from build123d import *

# Parameters (mm, degrees)
SKETCH1_R           = 10
BOSS_EXTRUDE1_DEPTH = 10


with BuildPart() as part:
    # Sketch1 → Boss-Extrude1 (new body)
    with BuildSketch(Plane.XY):
        Polygon((322.382476836, -17.859318996), (322.382476836, 42.140681004), (371.94488009, 42.140681004), (371.94488009, 332.140681004), (277.025034275, 332.140681004), (169.187054595, 271.975052979), (169.187054595, 205.170044114), (169.187054595, -17.859318996), align=None)
        with Locations((229.870255563, 265.671146953)):
            Circle(SKETCH1_R, mode=Mode.SUBTRACT)
        with Locations((229.870255563, 102.825256229)):
            Circle(SKETCH1_R, mode=Mode.SUBTRACT)
        with Locations((340.159565259, 299.323240315)):
            Circle(SKETCH1_R, mode=Mode.SUBTRACT)
        with Locations((340.159565259, 67.667528684)):
            Circle(SKETCH1_R, mode=Mode.SUBTRACT)
        with BuildLine():
            Line((312.226028305, 265.671146953), (312.226028305, 115.671146953))
            ThreePointArc((312.226028305, 115.671146953), (288.591642629, 92.036761277), (264.957256952, 115.671146953))
            Line((264.957256952, 115.671146953), (264.957256952, 265.671146953))
            ThreePointArc((264.957256952, 265.671146953), (288.591642629, 289.30553263), (312.226028305, 265.671146953))
        make_face(mode=Mode.SUBTRACT)
    extrude(amount=BOSS_EXTRUDE1_DEPTH)


solid = part.part
Input: part model. Units: mm. Frame: model coordinates. A direction names the side the tool comes from. Give positions to 0.01 mm unless a question says otherwise; leave off trailing zeros. Write each loop counter-clockwise with the first axis right and the second up, starting at its lowest first coordinate (ties: lowest second). Pieces come first, ordered by that corner, then holes. Notation, with made-up numbers: (2.25, -29.5) -> (16.25, -29.5) arc R22 cw to (16.25, -16.5) -> close; hole circle Ø5 at (-21.5, 57.25). An arc over 180 degrees is marked (long way). Use one line per item in the form item = value. Start each with the question number.
1) Draft query along X for faces 1 (the flat face through (169.187, 129, 5)), 2 (the cylindrical face through (239.41, 105.83, 4.93)), 3 (the flat face through (247, 160, 10)). Return one class per face: pulls with the +X half, pulls with the -X half, needs draft (parallel to the pull), parting line crosses it, or undercut.
2) Section query B-B on z = 6. Return the cut outline in (x, y).
3) Pin query (flat end, axial travel): pin 1 (3 mm diameter, centred on y = 8, z = 6.5, fed in from +X). Return the tip coordinate at first contact, or that it passes through.
4) Set-up query: faces 4 (the flat face through (347, 42.141, 5)), 5 (the flat face through (371.945, 185, 5)), 6 (the flat face through (312.226, 192, 5)). Return all of +Z, -Z, +X, -X, +Y, -Y with unobstructed straight access to the full face (end or side cutting, diameter ignored); none if empty.
5) Section query C-C on x = 235.5. Return the cut outline in (y, z), then the cut area to 3 significant figures.
6) Section query D-D on x = 308. Return the cut outline in (y, z).
7) Section query A-A on y = 196.5. Return the cut outline in (x, z), then the cut area to 3 significant figures.
8) Ray query, probe 1 along Y at (x, z) = (339, 3.5); probe 2 along X at (y, z) = (167.5, 1.5); probe 3 along Y at (x, z) = (224, 9.5). Return the intervals inside material, ascending. Write a range as from..to.
Outcome:
q1.face_1 = pulls with the -X half
q1.face_2 = undercut
q1.face_3 = needs draft
q2.outline = (169.19, -17.86) -> (322.38, -17.86) -> (322.38, 42.14) -> (371.94, 42.14) -> (371.94, 332.14) -> (277.03, 332.14) -> (169.19, 271.98) -> close; hole circle Ø20 at (229.87, 102.83); hole circle Ø20 at (229.87, 265.67); hole (264.96, 115.67) arc R23.63 ccw to (312.23, 115.67) -> (312.23, 265.67) arc R23.63 ccw to (264.96, 265.67) -> close; hole circle Ø20 at (340.16, 67.67); hole circle Ø20 at (340.16, 299.32)
q3.pin_1 = 322.38
q4.face_4 = +Z, -Z, +X, -Y
q4.face_5 = +Z, -Z, +X, +Y, -Y
q4.face_6 = +Z, -Z
q5.outline = (-17.86, 0) -> (94.56, 0) -> (94.56, 10) -> (-17.86, 10) -> close; (111.09, 0) -> (257.41, 0) -> (257.41, 10) -> (111.09, 10) -> close; (273.94, 0) -> (308.97, 0) -> (308.97, 10) -> (273.94, 10) -> close
q5.area = 2,940 mm^2
q6.outline = (-17.86, 0) -> (102.18, 0) -> (102.18, 10) -> (-17.86, 10) -> close; (279.16, 0) -> (332.14, 0) -> (332.14, 10) -> (279.16, 10) -> close
q7.outline = (169.19, 0) -> (264.96, 0) -> (264.96, 10) -> (169.19, 10) -> close; (312.23, 0) -> (371.94, 0) -> (371.94, 10) -> (312.23, 10) -> close
q7.area = 1,550 mm^2
q8.probe_1 = 42.14..57.73, 77.6..289.39, 309.26..332.14
q8.probe_2 = 169.19..264.96, 312.23..371.94
q8.probe_3 = -17.86..94.73, 110.92..257.58, 273.77..302.56
